Design review of the part built by this model. Coordinates are the model's own, in mm. A direction names the side the tool comes from. Round coordinates to 2 decimals unless told otherwise and drop trailing zeros. Write each loop counter-clockwise with the first axis right and the second up, starting at its lowest first coordinate (ties: lowest second). Pieces come first, ordered by that corner, then holes. Notation, with made-up numbers: (49.5, 58.5) -> (86.5, 58.5) arc R19 ccw to (86.5, 73.5) -> close; hole circle Ø5 at (69.25, -27.75). An arc over 180 degrees is marked (long way). One line per question, with ' | ' between items. Start each with the question number.
1) Consider section D-D (z = -7.25). Give the boundary of the cut face in (x, y) (1 decimal).
2) For probe 1 along Y at (x, z) = (0, -6.65); probe 2 along Y at (x, z) = (-1, -2.5), list the stretches that pass through material, from the lowest coordinate up.
3) Mouldability with a two-part tool opening along X and no side actions: class faces 4 (the cylindrical face through (-2.539, -1.947, -6.662)), 5 (the cylindrical face through (0.34, -1.55, -6.94)), 6 (the flat face through (0, -2, 0)) as +X half, -X half, draft (parallel to the pull), parting line (faces both ways), or undercut.
4) Consider section B-B (z = -0.75). Give the boundary of the cut face in (x, y).
5) For faces 1 (the flat face through (1.613, 0, -11)), 2 (the flat face through (0, -2, -13.5)), 3 (the flat face through (-1.613, 0, -3)), list the 3-axis set-ups (+Z, -Z, +X, -X, +Y, -Y) from which the entire face can be reached by the end or side of a thin tool; tool diameter is ignored.
Autodesk Inventor part; units mm, degrees
ref_plane "YZ Plane" through (0, 0, 0) normal (1, 0, 0) x (0, 1, 0)
ref_plane "XZ Plane" through (0, 0, 0) normal (0, 1, 0) x (-1, 0, 0)
ref_plane "XY Plane" through (0, 0, 0) normal (0, 0, 1) x (1, 0, 0)
sketch "Sketch1" plane through (0, 0, 0) normal (0, 0, 1) x (1, 0, 0)
  circle A0 centre (0, 0) radius 3.2
  dimension "d0" = 6.4
extrude "Extrusion1" add sketch "Sketch1" against normal blind 13.5
sketch "Sketch2" plane through (0, 0, 0) normal (0, 0, 1) x (1, 0, 0)
  circle A0 centre (0, 0) radius 2.7
  line L0 (1.6129, -1.5129) -> (1.6129, 1.5129)
  arc A1 (1.5129, -1.6129) -> (1.6129, -1.5129) centre (1.5129, -1.5129) ccw
  line L1 (-1.5129, -1.6129) -> (1.5129, -1.6129)
  arc A2 (-1.6129, -1.5129) -> (-1.5129, -1.6129) centre (-1.5129, -1.5129) ccw
  line L2 (-1.6129, 1.5129) -> (-1.6129, -1.5129)
  arc A3 (-1.5129, 1.6129) -> (-1.6129, 1.5129) centre (-1.5129, 1.5129) ccw
  line L3 (1.5129, 1.6129) -> (-1.5129, 1.6129)
  arc A4 (1.6129, 1.5129) -> (1.5129, 1.6129) centre (1.5129, 1.5129) ccw
extrude "Extrusion2" cut sketch "Sketch2" against normal blind 5.75 contours A1 L1 A2 L2 A3 L3 A4 L0
sketch "Sketch3" plane through (0, 0, -13.5) normal (0, 0, -1) x (-1, 0, 0)
  circle A0 centre (0, 0) radius 2.7
  line L0 (1.6129, -1.5129) -> (1.6129, 1.5129)
  arc A1 (1.5129, -1.6129) -> (1.6129, -1.5129) centre (1.5129, -1.5129) ccw
  line L1 (-1.5129, -1.6129) -> (1.5129, -1.6129)
  arc A2 (-1.6129, -1.5129) -> (-1.5129, -1.6129) centre (-1.5129, -1.5129) ccw
  line L2 (-1.6129, 1.5129) -> (-1.6129, -1.5129)
  arc A3 (-1.5129, 1.6129) -> (-1.6129, 1.5129) centre (-1.5129, 1.5129) ccw
  line L3 (1.5129, 1.6129) -> (-1.5129, 1.6129)
  arc A4 (1.6129, 1.5129) -> (1.5129, 1.6129) centre (1.5129, 1.5129) ccw
extrude "Extrusion3" cut sketch "Sketch3" against normal blind 5.4 contours A1 L1 A2 L2 A3 L3 A4 L0
sketch "Sketch4" plane through (0, 0, -8.1) normal (0, 0, -1) x (-1, 0, 0)
  circle A0 centre (0, 0) radius 1.5875
  dimension "d7" = 3.175
extrude "Extrusion4" cut sketch "Sketch4" against normal up to next
chamfer "Chamfer1" distance 0.5 angle 45 2 edges at (-3.2, 0, -13.5) (-3.2, 0, 0)
sketch "Sketch5" plane through (0, 0, 0) normal (0, 0, 1) x (1, 0, 0)
  line L0 (1.6129, 1.5129) -> (1.6129, -1.5129)
  line L1 (1.5129, -1.6129) -> (-1.5129, -1.6129)
  line L2 (-1.6129, -1.5129) -> (-1.6129, 1.5129)
  line L3 (-1.5129, 1.6129) -> (1.5129, 1.6129)
  circle A0 centre (0, 0) radius 2.7
  circle A1 centre (0, 0) radius 1.6129
surface extrude "ExtrusionSrf1" sketch "Sketch5" against normal up to surface (13.5 mm away) shown no curves A1
properties part number "276-1843" material "Steel"
From the geometry:
1) outline: circle Ø6.4 at (0, 0); hole circle Ø3.2 at (0, 0)
2) probe 1: y = -3.2 to -1.59, 1.59 to 3.2 | probe 2: y = -3.04 to -1.61, 1.61 to 3.04
3) face 4: parting line | face 5: undercut | face 6: draft
4) outline: circle Ø6.4 at (0, 0); hole (-1.61, -1.51) arc R0.1 ccw to (-1.51, -1.61) -> (1.51, -1.61) arc R0.1 ccw to (1.61, -1.51) -> (1.61, 1.51) arc R0.1 ccw to (1.51, 1.61) -> (-1.51, 1.61) arc R0.1 ccw to (-1.61, 1.51) -> close
5) face 1: -Z | face 2: -Z, +X, -X, +Y, -Y | face 3: +Z
